```python
from build123d import *

# Parameters (mm, degrees)
F0_W     = 30
F0_H     = 30
F1_DEPTH = 4
F2_T     = -4
F3_R     = 1
F4_R     = 4
F5_R     = 1


with BuildPart() as f1:
    # F0 (on Top) → F1 (new body)
    with BuildSketch(Plane.XY):
        Rectangle(F0_W, F0_H)
    extrude(amount=F1_DEPTH)

    # F2
    f2_openings = [f1.faces().sort_by_distance(p)[0] for p in [
        (0, 0, 4),
        (0, 0, 0),
    ]]
    offset(amount=F2_T, openings=f2_openings)

    # F3
    f3_edges = [f1.edges().sort_by_distance(p)[0] for p in [
        (-11, 11, 2),
        (11, 11, 2),
        (-11, -11, 2),
        (11, -11, 2),
    ]]
    fillet(f3_edges, radius=F3_R)

    # F4
    f4_edges = [f1.edges().sort_by_distance(p)[0] for p in [
        (-15, 15, 2),
        (15, 15, 2),
        (-15, -15, 2),
        (15, -15, 2),
    ]]
    fillet(f4_edges, radius=F4_R)

    # F5
    f5_edges = [f1.edges().sort_by_distance(p)[0] for p in [
        (11, 0, 4),
        (15, 0, 4),
        (13.828427, 13.828427, 0),
        (10.707107, 10.707107, 0),
    ]]
    fillet(f5_edges, radius=F5_R)


solid = f1.part
```
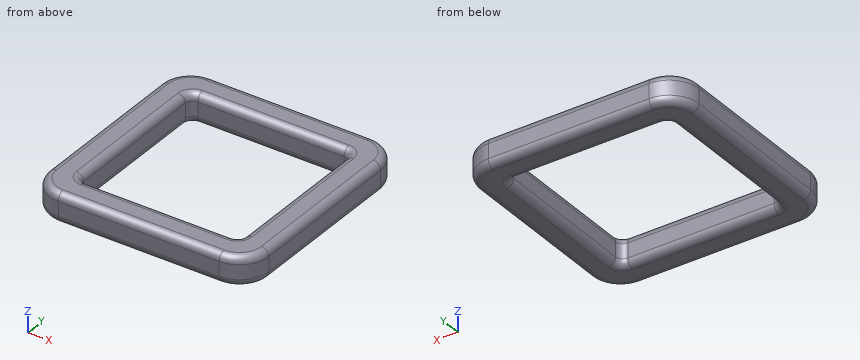
Verification items for the finished model (mm, model axes). Round coordinates to 2 decimals unless told otherwise and drop trailing zeros. Order: outer loops, then holes, each group sorted by start corner. A loop starts at its lowest first (then second) coordinate and runs counter-clockwise, first axis right, second up. Notation, with made-up numbers: (70.25, 42.25) - (101.25, 42.25) arc R26 ccw to (101.25, 64.25) - close; hole circle Ø3 at (58.25, -31.5). An arc over 180 degrees is marked (long way). Use CSV: the item, a comma, the result in double quotes.
(1) Section check A-A on y = -1.5. Record the boundary of the cut face in (x, z), and give its area (3 significant figures).
Entries:
outline,"(-15, 1) arc R1 ccw to (-14, 0) - (-12, 0) arc R1 ccw to (-11, 1) - (-11, 3) arc R1 ccw to (-12, 4) - (-14, 4) arc R1 ccw to (-15, 3) - close; (11, 1) arc R1 ccw to (12, 0) - (14, 0) arc R1 ccw to (15, 1) - (15, 3) arc R1 ccw to (14, 4) - (12, 4) arc R1 ccw to (11, 3) - close"
area,"30.3 mm^2"
(2) Section check B-B on z = 1.4. Record the boundary of the cut face in (x, y).
Entries:
outline,"(-15, -11) arc R4 ccw to (-11, -15) - (11, -15) arc R4 ccw to (15, -11) - (15, 11) arc R4 ccw to (11, 15) - (-11, 15) arc R4 ccw to (-15, 11) - close; hole (-11, -10) arc R1 ccw to (-10, -11) - (10, -11) arc R1 ccw to (11, -10) - (11, 10) arc R1 ccw to (10, 11) - (-10, 11) arc R1 ccw to (-11, 10) - close"
(3) Thickness scan on probe 1 along X at (y, z) = (2.25, 1.9); probe 2 along Y at (x, z) = (-8, 3.5). Record the ranges inside material, lowest first. Write a range as from..to.
Entries:
probe 1,"-15..-11, 11..15"
probe 2,"-14.87..-11.13, 11.13..14.87"
(4) Section check D-D on z = 3.5. Record the boundary of the cut face in (x, y).
Entries:
outline,"(-14.87, -11) arc R3.87 ccw to (-11, -14.87) - (11, -14.87) arc R3.87 ccw to (14.87, -11) - (14.87, 11) arc R3.87 ccw to (11, 14.87) - (-11, 14.87) arc R3.87 ccw to (-14.87, 11) - close; hole (-11.13, -10) arc R1.13 ccw to (-10, -11.13) - (10, -11.13) arc R1.13 ccw to (11.13, -10) - (11.13, 10) arc R1.13 ccw to (10, 11.13) - (-10, 11.13) arc R1.13 ccw to (-11.13, 10) - close"
